Source: three-view drawing plus pictorial views. Frame: mm from the lowest corner of the part. A direction names the side the tool comes from. Give positions to 0.01 mm unless a question says otherwise; leave off trailing zeros. Loops run counter-clockwise (first coordinate to the right, second up) from the corner with the lowest first, then second, coordinate; pieces in that order, holes last.
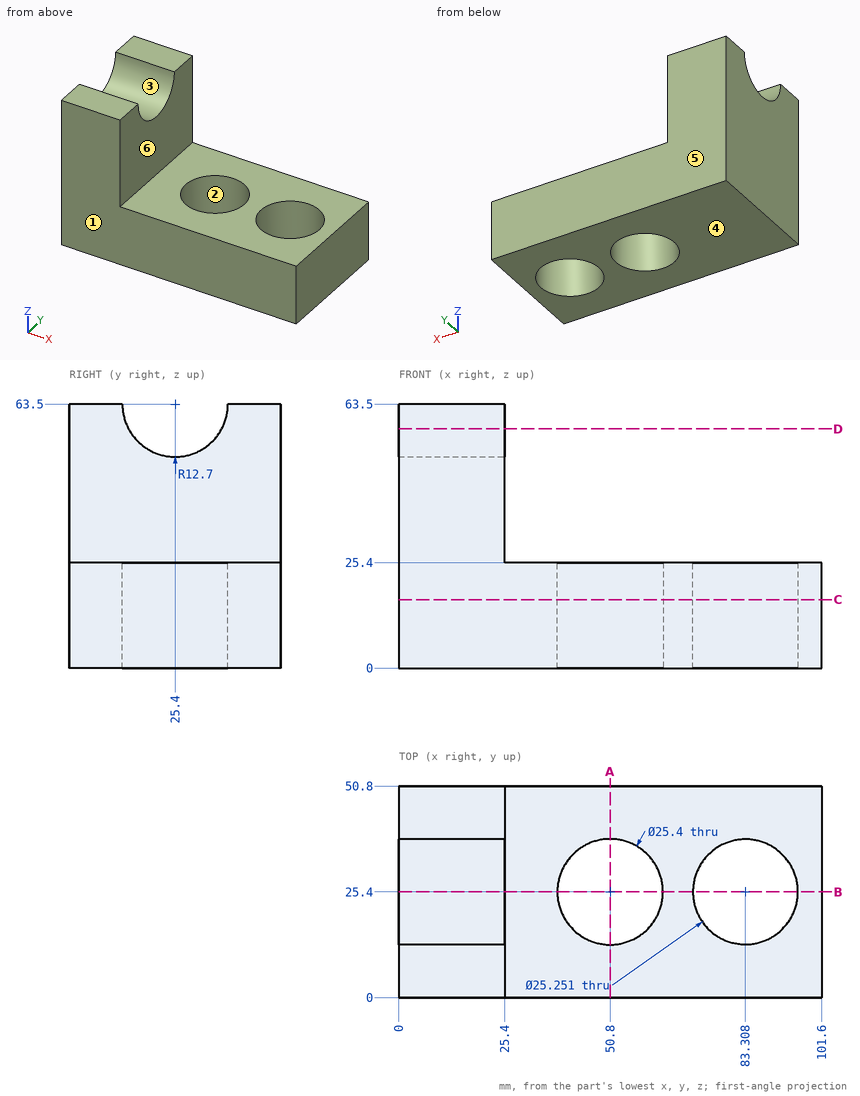
1) Cut plane A-A (x = 50.8). Return loops of the section in (y, z), and give its area (3 significant figures).
Checks:
outline: (0, 0) - (12.7, 0) - (12.7, 25.4) - (0, 25.4) - close; (38.1, 0) - (50.8, 0) - (50.8, 25.4) - (38.1, 25.4) - close
area: 645 mm2
2) Ray query, probe 1 along X at (y, z) = (25, 7); probe 2 along X at (y, z) = (14, 26). Return the intervals inside material, ascending.
Checks:
probe 1: x = 0 to 38.11, 63.49 to 70.69, 95.93 to 101.6
probe 2: x = 0 to 25.4
3) Contact query for flat-ended pins moving along their axis: P1, Ø1, axis at y = 23.5, z = 44, coming from the +X side; P2, Ø15, axis at x = 83.31, y = 25.4, coming from the +Z side. Output: stop coordinate, or through.
Checks:
P1: stops at x = 25.4
P2: passes through
4) Reachability of the marked faces 5 and 6 from +Z, -Z, +X, -X, +Y, -Y: full face, straight path, thin tool, end or side. Return the list, or none.
Checks:
face 5: +Z, -Z, +X, -X, +Y
face 6: +Z, +X, +Y, -Y
5) Cut plane D-D (z = 57.5). Return loops of the section in (x, y).
Checks:
outline: (0, 0) - (25.4, 0) - (25.4, 14.21) - (0, 14.21) - close; (0, 36.59) - (25.4, 36.59) - (25.4, 50.8) - (0, 50.8) - close
6) Cut plane C-C (z = 16.5). Return loops of the section in (x, y) (1 decimal), and give its area (3 significant figures).
Checks:
outline: (0, 0) - (101.6, 0) - (101.6, 50.8) - (0, 50.8) - close; hole circle Ø25.4 at (50.8, 25.4); hole circle Ø25.3 at (83.3, 25.4)
area: 4,150 mm2
7) Pull-direction query (Y, two-part tool) for the marked faces 1, 2, 3 and 4; classes: released by +Y, released by -Y, zero draft, split by the parting line, or undercut.
Checks:
face 1: released by -Y
face 2: undercut
face 3: undercut
face 4: zero draft
8) Cut plane B-B (y = 25.4). Return loops of the section in (x, z) (1 decimal), and give its area (3 significant figures).
Checks:
outline: (0, 0) - (38.1, 0) - (38.1, 25.4) - (25.4, 25.4) - (25.4, 50.8) - (0, 50.8) - close; (63.5, 0) - (70.7, 0) - (70.7, 25.4) - (63.5, 25.4) - close; (95.9, 0) - (101.6, 0) - (101.6, 25.4) - (95.9, 25.4) - close
area: 1,940 mm2
